Source: CAD feature listing. Evaluate the final solid. Frame: model axes, mm. Round coordinates to 2 decimals unless told otherwise and drop trailing zeros. Put each result on its own line as item: value.
```python
from build123d import *

# Parameters (mm, degrees)
SKETCH1_R           = 3.2385
BOSS_EXTRUDE1_DEPTH = 2.54


with BuildPart() as part:
    # Sketch1 → Boss-Extrude1 (new body)
    with BuildSketch(Plane(origin=(0, 0, 0), x_dir=(1, 0, 0), z_dir=(0, 1, 0))):
        Polygon((123.825, 152.4), (123.825, 123.825), (152.4, 123.825), (152.4, -123.825), (123.825, -123.825), (123.825, -152.4), (-123.825, -152.4), (-123.825, -123.825), (-152.4, -123.825), (-152.4, 123.825), (-123.825, 123.825), (-123.825, 152.4), align=None)
        with Locations((76.2, 139.7)):
            Circle(SKETCH1_R, mode=Mode.SUBTRACT)
        with Locations((0, 139.7)):
            Circle(SKETCH1_R, mode=Mode.SUBTRACT)
        with Locations((-76.2, 139.7)):
            Circle(SKETCH1_R, mode=Mode.SUBTRACT)
        with Locations((-76.2, -139.7)):
            Circle(SKETCH1_R, mode=Mode.SUBTRACT)
        with Locations((0, -139.7)):
            Circle(SKETCH1_R, mode=Mode.SUBTRACT)
        with Locations((76.2, -139.7)):
            Circle(SKETCH1_R, mode=Mode.SUBTRACT)
        with Locations((139.7, -76.2)):
            Circle(SKETCH1_R, mode=Mode.SUBTRACT)
        with Locations((139.7, 0)):
            Circle(SKETCH1_R, mode=Mode.SUBTRACT)
        with Locations((139.7, 76.2)):
            Circle(SKETCH1_R, mode=Mode.SUBTRACT)
        with Locations((-139.7, 76.2)):
            Circle(SKETCH1_R, mode=Mode.SUBTRACT)
        with Locations((-139.7, 0)):
            Circle(SKETCH1_R, mode=Mode.SUBTRACT)
        with Locations((-139.7, -76.2)):
            Circle(SKETCH1_R, mode=Mode.SUBTRACT)
    extrude(amount=BOSS_EXTRUDE1_DEPTH)


solid = part.part
```
Q1. Cut plane A-A on y = 1.6. Give the number of separate pieces and of enclosed holes in the cut face, and give its area (3 significant figures).
Ans:
separate pieces: 1
enclosed holes: 12
area: 89,200 mm^2
Q2. Material intervals for line 1 (Z direction, x = 139.7, y = 1.75) (1 decimal); line 2 (Z direction, x = 0, y = 1.1), sorted ascending. Write a range as [from, to].
Ans:
line 1: z = [-123.8, -79.4], [-73, -3.2], [3.2, 73], [79.4, 123.8]
line 2: z = [-152.4, -142.94], [-136.46, 136.46], [142.94, 152.4]
Q3. Draft query along Z for faces 1 (the cylindrical face through (136.465, 1.252, -76.342)), 2 (the cylindrical face through (1.494, 1.252, 142.573)), 3 (the flat face through (2, 0, -2)). Return one class per face: +Z half, -Z half, draft (parallel to the pull), parting line (faces both ways), or undercut.
Ans:
face 1: undercut
face 2: undercut
face 3: draft
Q4. Pin query (flat end, axial travel): pin 1 (1.3 mm diameter, centred on x = -143.5, y = 1.5, fed in from +Z) (3 decimals); pin 2 (0.8 mm diameter, centred on x = -144, y = 2, fed in from -Z) (3 decimals); pin 3 (4 mm diameter, centred on x = 139.7, z = -76.2, fed in from +Y). Return the tip coordinate at first contact, or that it passes through.
Ans:
pin 1: stops at z = 123.825
pin 2: stops at z = -123.825
pin 3: passes through
